from build123d import *

# Parameters (mm, degrees)
BOSS_EXTRUDE1_DEPTH         = 12.5
BOSS_EXTRUDE1_DEPTH_BACK    = 12.5
SKETCH4_R                   = 2
CUT_EXTRUDE2_DEPTH          = 31.409702399
CUT_EXTRUDE3_REACH          = 32.899
SKETCH7_R                   = 5
TAP_DRILL_FOR_M3X0_5_TAP2_D = 2.5


with BuildPart() as part:
    # Sketch2 → Boss-Extrude1 (new, two sides: drawn at the far end of the back side and taken through both)
    with BuildSketch(Plane(origin=(0, 0, 0), x_dir=(0, 0, -1), z_dir=(1, 0, 0)).offset(-BOSS_EXTRUDE1_DEPTH_BACK)):
        Polygon((0, 0), (27.5, 0), (27.5, 3), (12.5, 3), (12.5, 6.5), (-12.5, 6.5), (-12.5, 3), (-27.5, 3), (-27.5, 0), align=None)
    extrude(amount=BOSS_EXTRUDE1_DEPTH + BOSS_EXTRUDE1_DEPTH_BACK)

    # Sketch4 → Cut-Extrude2 (cut, through all)
    with BuildSketch(Plane(origin=(0, 3, 0), x_dir=(1, 0, 0), z_dir=(0, 1, 0))):
        with Locations(Location((-8.5, 20, 0), (0, 0, 270))):
            Circle(SKETCH4_R)
        with Locations(Location((8.5, 20, 0), (0, 0, 90))):
            Circle(SKETCH4_R)
        with Locations(Location((8.5, -20, 0), (0, 0, 270))):
            Circle(SKETCH4_R)
        with Locations(Location((-8.5, -20, 0), (0, 0, 90))):
            Circle(SKETCH4_R)
    extrude(amount=-CUT_EXTRUDE2_DEPTH, mode=Mode.SUBTRACT)

    # Sketch7 → Cut-Extrude3 (cut, up to next)
    with BuildSketch(Plane(origin=(0, 6.5, 0), x_dir=(1, 0, 0), z_dir=(0, 1, 0)), mode=Mode.PRIVATE) as cut_extrude3_sk1:
        with Locations(Location((0, 0, 0), (0, 0, 270))):
            Circle(SKETCH7_R)
    cut_extrude3_tool1 = extrude(cut_extrude3_sk1.sketch, amount=-CUT_EXTRUDE3_REACH, mode=Mode.PRIVATE) & part.part
    add(cut_extrude3_tool1.solids().sort_by_distance((0, 6.5, 0))[0], mode=Mode.SUBTRACT)

    # Tap Drill for M3x0.5 Tap2 (through all)
    with Locations(Plane(origin=(0, 6.5, 0), x_dir=(1, 0, 0), z_dir=(0, 1, 0))):
        with Locations((0, 9.53), (0, -9.53)):
            Hole(TAP_DRILL_FOR_M3X0_5_TAP2_D / 2)


solid = part.part
For this review, take the finished solid that the model builds, in its own axes (mm). A direction names the side the tool comes from. Give positions to 0.01 mm unless a question says otherwise; leave off trailing zeros. Loops run counter-clockwise (first coordinate to the right, second up) from the corner with the lowest first, then second, coordinate; pieces in that order, holes last. Notation, with made-up numbers: M 11,-12 L 23,-12 A3 cw 23,-8 Z; hole C 69.5,54.5 d6. An arc over 180 degrees is marked long. Answer as a JSON object with one key per item and string values. Group by question number.
Q1. Insertion check: P1, Ø7.5, axis at x = 1.5, z = 17, coming from the +Y side; P2, Ø1.8, axis at x = 2.5, y = 5, coming from the +Z side. Each pin has a flat end and moves straight along its axis. Give the tip position at first contact, or say it passes through.
Q2. Add section D-D on x = 8.5. Give the boundary of the cut face in (y, z).
Q3. Add section C-C on y = 5. Give the boundary of the cut face in (x, z), and give its area (3 significant figures).
Q4. Mouldability with a two-part tool opening along X and no side actions: class faces 4 (the cylindrical face through (-0.577, 3.204, -8.421)), 5 (the flat face through (12.5, 3, 0)), 6 (the cylindrical face through (-4.88, 3.3, -1.08)), 7 (the flat face through (0, 3, -20)) as +X half, -X half, draft (parallel to the pull), parting line (faces both ways), or undercut.
Q5. Tool access review of faces 1 (the flat face through (0, 5, -12.5)), 2 (the cylindrical face through (9.852, 1.521, 18.526)), 3 (the flat face through (0, 3, 20)): name each direction out of +Z, -Z, +X, -X, +Y, -Y from which nothing blocks a thin tool from reaching the whole face with its end or side.
Q6. For probe 1 along X at (y, z) = (1.9, 20); probe 2 along Y at (x, z) = (6.5, -19); probe 3 along X at (y, z) = (3, -0.5), list the stretches that pass through material, from the lowest coordinate up. Write a range as [from, to].
Q7. Add section B-B on x = 0. Give the boundary of the cut face in (y, z).
Q8. Add section A-A on z = 9.53. Give the boundary of the cut face in (x, y).
Checked values:
{
 "1": {"P1": "y = 3", "P2": "z = 12.5"},
 "2": {"outline": "M 0,-27.5 L 3,-27.5 L 3,-22 L 0,-22 Z; M 0,-18 L 3,-18 L 3,-12.5 L 6.5,-12.5 L 6.5,12.5 L 3,12.5 L 3,18 L 0,18 Z; M 0,22 L 3,22 L 3,27.5 L 0,27.5 Z"},
 "3": {"outline": "M -12.5,-12.5 L 12.5,-12.5 L 12.5,12.5 L -12.5,12.5 Z; hole C 0,0 d10; hole C 0,-9.53 d2.5; hole C 0,9.53 d2.5", "area": "537 mm²"},
 "4": {"face 4": "undercut", "face 5": "+X half", "face 6": "undercut", "face 7": "draft"},
 "5": {"face 1": "-Z, +X, -X, +Y", "face 2": "+Y, -Y", "face 3": "+Z, +X, -X, +Y"},
 "6": {"probe 1": "[-12.5, -10.5], [-6.5, 6.5], [10.5, 12.5]", "probe 2": "[0, 3]", "probe 3": "[-12.5, -4.97], [4.97, 12.5]"},
 "7": {"outline": "M 0,-27.5 L 3,-27.5 L 3,-12.5 L 6.5,-12.5 L 6.5,-10.78 L 0,-10.78 Z; M 0,-8.28 L 6.5,-8.28 L 6.5,-5 L 0,-5 Z; M 0,5 L 6.5,5 L 6.5,8.28 L 0,8.28 Z; M 0,10.78 L 6.5,10.78 L 6.5,12.5 L 3,12.5 L 3,27.5 L 0,27.5 Z"},
 "8": {"outline": "M -12.5,0 L -1.25,0 L -1.25,6.5 L -12.5,6.5 Z; M 1.25,0 L 12.5,0 L 12.5,6.5 L 1.25,6.5 Z"}
}
